Part model, mm, in its own coordinate system. A direction names the side the tool comes from. Coordinates: 2 decimals unless noted, no trailing zeros. Loops run counter-clockwise (first coordinate to the right, second up) from the corner with the lowest first, then second, coordinate; pieces in that order, holes last. Notation, with made-up numbers: (-26.75, -14.75) - (25.25, -14.75) arc R7 ccw to (25.25, -6.75) - close; hole circle Ø1 at (52.5, 0). An arc over 180 degrees is marked (long way). Use a Markdown table: item, result. Add a question column.
1. Drop flat-ended pins along their axis: pin 1 (12 mm diameter, centred on x = 18.5, y = 38, fed in from +Z); pin 2 (3.5 mm diameter, centred on y = 9.5, z = 13, fed in from +X); pin 3 (4 mm diameter, centred on x = -25.5, z = 5, fed in from -Y); pin 4 (3 mm diameter, centred on x = 13.5, z = 3, fed in from -Y). Give the stop position or say it passes through.
2. 3-axis set-ups, long thin cutter, end or side, ignore diameter. For faces 4 (the flat face through (-20, 8, 14)), 5 (the flat face through (30, 8, 5)), 6 (the flat face through (-13, 40.8, 5.1)), 7 (the flat face through (26, 20, 5)): which of +Z, -Z, +X, -X, +Y, -Y reach the whole face in a straight line?
3. Band-saw the part on D-D, the plane x = 0. Give the cut face in (y, z), plus the area to 3 significant figures.
4. Wall check: probe 1 along Y at (x, z) = (21.5, 4.5); probe 2 along Y at (x, z) = (-24.75, 12); probe 3 along Z at (x, y) = (25.5, 8.25). Give the ranges that are in metal, low to high. Write a range as [from, to].
5. Pull direction Y, two halves, no side cores. Call faces 1 (the flat face through (-11.8, 27, 5)), 2 (the flat face through (-23.8, 0, 3.8)), 3 (the cylindrical face through (27.25, 8.11, 5.08)): pulls with the +Y half, pulls with the -Y half, needs draft (parallel to the pull), parting line crosses it, or undercut.
6. Band-saw the part on C-C, the plane y = 44. Give the cut face in (x, z), plus the area to 3 significant figures.
7. Band-saw the part on B-B, the plane z = 5. Count the separate pieces of the cut face and the enclosed holes in it, plus the area to 3 significant figures.
8. Band-saw the part on A-A, the plane x = 25.5. Give the cut face in (y, z).
from build123d import *

# Parameters (mm, degrees)
Y_KSEKLIK_EKSTR_ZYON1_DEPTH = 10
CUT_EXTRUDE1_REACH          = 62.86
SKETCH1_W                   = 10
SKETCH1_H                   = 4
SKETCH1_H_2                 = 36
CUT_EXTRUDE2_REACH          = 49.917
SKETCH2_R                   = 1.75
SKETCH3_W                   = 10
SKETCH3_H                   = 10
BOSS_EXTRUDE1_DEPTH         = 7
CUT_EXTRUDE3_REACH          = 83.197
SKETCH4_R                   = 1.5
CUT_EXTRUDE4_REACH          = 62.86
CUT_EXTRUDE5_REACH          = 73.851
SKETCH7_R                   = 4.5
SKETCH8_W                   = 10
SKETCH8_H                   = 32
BOSS_EXTRUDE2_DEPTH         = 3


with BuildPart() as part:
    # Çizim1 → Yükseklik-Ekstrüzyon1 (new body)
    with BuildSketch(Plane.XY):
        with BuildLine():
            Line((-30, 0), (-17.5, 0))
            ThreePointArc((-17.5, 0), (0, 17.5), (17.5, 0))
            Line((17.5, 0), (30, 0))
            Line((30, 0), (30, 52))
            Line((30, 52), (-30, 52))
            Line((-30, 52), (-30, 0))
        make_face()
    extrude(amount=Y_KSEKLIK_EKSTR_ZYON1_DEPTH)

    # Sketch1 → Cut-Extrude1 (cut, up to next)
    with BuildSketch(Plane.XY.offset(10), mode=Mode.PRIVATE) as cut_extrude1_sk1:
        with Locations((25, 18)):
            Rectangle(SKETCH1_W, SKETCH1_H)
    cut_extrude1_tool1 = extrude(cut_extrude1_sk1.sketch, amount=-CUT_EXTRUDE1_REACH, mode=Mode.PRIVATE) & part.part
    # Sketch1 → Cut-Extrude1 (cut, up to next)
    with BuildSketch(Plane.XY.offset(10), mode=Mode.PRIVATE) as cut_extrude1_sk2:
        with Locations((-25, 34)):
            Rectangle(SKETCH1_W, SKETCH1_H_2)
    cut_extrude1_tool2 = extrude(cut_extrude1_sk2.sketch, amount=-CUT_EXTRUDE1_REACH, mode=Mode.PRIVATE) & part.part
    add(cut_extrude1_tool1.solids().sort_by_distance((25, 18, 10))[0], mode=Mode.SUBTRACT)
    add(cut_extrude1_tool2.solids().sort_by_distance((-25, 34, 10))[0], mode=Mode.SUBTRACT)

    # Sketch2 → Cut-Extrude2 (cut, up to next)
    with BuildSketch(Plane(origin=(0, 16, 0), x_dir=(1, 0, 0), z_dir=(0, 1, 0)), mode=Mode.PRIVATE) as cut_extrude2_sk1:
        with Locations(Location((-25.5, -5, 0), (0, 0, 180))):
            Circle(SKETCH2_R)
    cut_extrude2_tool1 = extrude(cut_extrude2_sk1.sketch, amount=-CUT_EXTRUDE2_REACH, mode=Mode.PRIVATE) & part.part
    # Sketch2 → Cut-Extrude2 (cut, up to next)
    with BuildSketch(Plane(origin=(0, 16, 0), x_dir=(1, 0, 0), z_dir=(0, 1, 0)), mode=Mode.PRIVATE) as cut_extrude2_sk2:
        with Locations(Location((25.5, -5, 0), (0, 0, 180))):
            Circle(SKETCH2_R)
    cut_extrude2_tool2 = extrude(cut_extrude2_sk2.sketch, amount=-CUT_EXTRUDE2_REACH, mode=Mode.PRIVATE) & part.part
    add(cut_extrude2_tool1.solids().sort_by_distance((-25.5, 16, 5))[0], mode=Mode.SUBTRACT)
    add(cut_extrude2_tool2.solids().sort_by_distance((25.5, 16, 5))[0], mode=Mode.SUBTRACT)

    # Sketch3 → Boss-Extrude1 (add)
    with BuildSketch(Plane.XY.offset(10)):
        with Locations((-25, 8)):
            Rectangle(SKETCH3_W, SKETCH3_H)
    extrude(amount=BOSS_EXTRUDE1_DEPTH)

    # Sketch4 → Cut-Extrude3 (cut, up to next)
    with BuildSketch(Plane.ZY.offset(30), mode=Mode.PRIVATE) as cut_extrude3_sk1:
        with Locations((12, 8)):
            Circle(SKETCH4_R)
    cut_extrude3_tool1 = extrude(cut_extrude3_sk1.sketch, amount=-CUT_EXTRUDE3_REACH, mode=Mode.PRIVATE) & part.part
    add(cut_extrude3_tool1.solids().sort_by_distance((-30, 8, 12))[0], mode=Mode.SUBTRACT)

    # Sketch6 → Cut-Extrude4 (cut, up to next)
    with BuildSketch(Plane.XY.offset(10), mode=Mode.PRIVATE) as cut_extrude4_sk1:
        with BuildLine():
            Line((-20, 52), (-16.579251378, 52))
            Line((-16.579251378, 52), (-16.579251378, 18))
            ThreePointArc((-16.579251378, 18), (-17.165037815, 16.585786438), (-18.579251378, 16))
            Line((-18.579251378, 16), (-20, 16))
            Line((-20, 16), (-20, 52))
        make_face()
    cut_extrude4_tool1 = extrude(cut_extrude4_sk1.sketch, amount=-CUT_EXTRUDE4_REACH, mode=Mode.PRIVATE) & part.part
    # Sketch6 → Cut-Extrude4 (cut, up to next)
    with BuildSketch(Plane.XY.offset(10), mode=Mode.PRIVATE) as cut_extrude4_sk2:
        Polygon((27.2, 45), (-11.8, 45), (-11.8, 42), (-14.3, 39.5), (-14.3, 30.5), (-11.8, 28), (-11.8, 25), (27.2, 25), align=None)
    cut_extrude4_tool2 = extrude(cut_extrude4_sk2.sketch, amount=-CUT_EXTRUDE4_REACH, mode=Mode.PRIVATE) & part.part
    add(cut_extrude4_tool1.solids().sort_by_distance((-18.298496, 34.123216, 10))[0], mode=Mode.SUBTRACT)
    add(cut_extrude4_tool2.solids().sort_by_distance((6.965585, 35, 10))[0], mode=Mode.SUBTRACT)

    # Sketch7 → Cut-Extrude5 (cut, up to next)
    with BuildSketch(Plane.ZY.offset(16.579251378), mode=Mode.PRIVATE) as cut_extrude5_sk1:
        with Locations((12, 35)):
            Circle(SKETCH7_R)
    cut_extrude5_tool1 = extrude(cut_extrude5_sk1.sketch, amount=-CUT_EXTRUDE5_REACH, mode=Mode.PRIVATE) & part.part
    add(cut_extrude5_tool1.solids().sort_by_distance((-16.579251, 35, 12))[0], mode=Mode.SUBTRACT)

    # Sketch8 → Boss-Extrude2 (add)
    with BuildSketch(Plane(origin=(30, 0, 0), x_dir=(0, 0, -1), z_dir=(1, 0, 0))):
        with Locations((-5, 36)):
            Rectangle(SKETCH8_W, SKETCH8_H)
    extrude(amount=BOSS_EXTRUDE2_DEPTH)


solid = part.part
Geometry check:
| question | item | result |
|---|---|---|
| 1 | pin 1 | passes through |
| 1 | pin 2 | stops at x = -20 |
| 1 | pin 3 | stops at y = 0 |
| 1 | pin 4 | stops at y = 9.01 |
| 2 | face 4 | +Z, +X, +Y, -Y |
| 2 | face 5 | +Z, -Z, +X, -Y |
| 2 | face 6 | +Z, -Z |
| 2 | face 7 | +Z, -Z, +X |
| 3 | outline | (17.5, 0) - (25, 0) - (25, 10) - (17.5, 10) - close; (45, 0) - (52, 0) - (52, 10) - (45, 10) - close |
| 3 | area | 145 mm^2 |
| 4 | probe 1 | y = [0, 16], [20, 25], [45, 52] |
| 4 | probe 2 | y = [3, 6.5], [9.5, 13] |
| 4 | probe 3 | z = [0, 3.25], [6.75, 10] |
| 5 | face 1 | undercut |
| 5 | face 2 | pulls with the -Y half |
| 5 | face 3 | needs draft |
| 6 | outline | (-16.58, 0) - (-11.8, 0) - (-11.8, 10) - (-16.58, 10) - close; (27.2, 0) - (33, 0) - (33, 10) - (27.2, 10) - close |
| 6 | area | 106 mm^2 |
| 7 | separate pieces | 3 |
| 7 | enclosed holes | 1 |
| 7 | area | 1,290 mm^2 |
| 8 | outline | (0, 0) - (16, 0) - (16, 3.25) - (0, 3.25) - close; (0, 6.75) - (16, 6.75) - (16, 10) - (0, 10) - close; (20, 0) - (25, 0) - (25, 10) - (20, 10) - close; (45, 0) - (52, 0) - (52, 10) - (45, 10) - close |
